```python
from build123d import *

# Parameters (mm, degrees)
SKETCH1_R             = 7.5
BOSS_EXTRUDE1_DEPTH   = 33
M6_TAPPED_HOLE1_D     = 5
M6_TAPPED_HOLE1_DEPTH = 16
M6_TAPPED_HOLE1_TIP   = 1.502151548
M6_TAPPED_HOLE2_D     = 5
M6_TAPPED_HOLE2_DEPTH = 16
M6_TAPPED_HOLE2_TIP   = 1.502151548


with BuildPart() as part:
    # Sketch1 → Boss-Extrude1 (new, symmetric)
    with BuildSketch(Plane.XY):
        Circle(SKETCH1_R)
    extrude(amount=BOSS_EXTRUDE1_DEPTH, both=True)

    # M6 Tapped Hole1
    with Locations(Plane.XY.offset(33)):
        with Locations((0, 0)):
            Hole(M6_TAPPED_HOLE1_D / 2, depth=M6_TAPPED_HOLE1_DEPTH)
            with Locations((0, 0, -(M6_TAPPED_HOLE1_DEPTH + M6_TAPPED_HOLE1_TIP / 2))):  # 118° drill point
                Cone(0, M6_TAPPED_HOLE1_D / 2, M6_TAPPED_HOLE1_TIP, mode=Mode.SUBTRACT)

    # M6 Tapped Hole2
    with Locations(Plane(origin=(0, 0, -33), x_dir=(-1, 0, 0), z_dir=(0, 0, -1))):
        with Locations((0, 0)):
            Hole(M6_TAPPED_HOLE2_D / 2, depth=M6_TAPPED_HOLE2_DEPTH)
            with Locations((0, 0, -(M6_TAPPED_HOLE2_DEPTH + M6_TAPPED_HOLE2_TIP / 2))):  # 118° drill point
                Cone(0, M6_TAPPED_HOLE2_D / 2, M6_TAPPED_HOLE2_TIP, mode=Mode.SUBTRACT)


solid = part.part
```
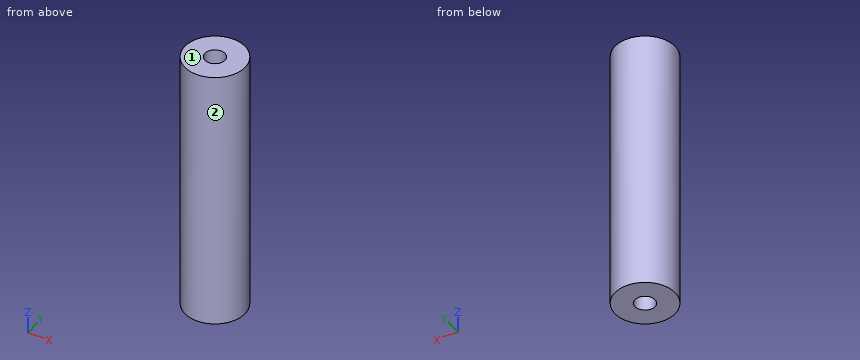
Here's how the part is built. I have some questions about the finished solid (model axes, mm). Face numbers are marked on the shaded views. Coordinates: 2 decimals unless noted, no trailing zeros. Order: outer loops, then holes, each group sorted by start corner. A loop starts at its lowest first (then second) coordinate and runs counter-clockwise, first axis right, second up. Notation, with made-up numbers: M -38,28.5 L 11,28.5 A20 ccw 11,63.5 Z; hole C 68.5,-38.5 d9. An arc over 180 degrees is marked long. Answer as a JSON object with one key per item and string values. Group by question number.
(1) If we mould it in two halves opening along X, with no side actions, what happens to the marked faces 1 and 2? For each: released by +X, released by -X, zero draft, split by the parting line, or undercut.
(2) Suppose I cut it at C-C, the plane x = -6. Please give me the cut outline in (y, z).
(3) Suppose I cut it at D-D, the plane y = 3.75. Please give me the cut outline in (x, z), then the cut area to 3 significant figures.
(4) Suppose I cut it at A-A, the plane z = 8. Please give me the cut outline in (x, y), then the cut area to 3 significant figures.
(5) I need wall thicknesses on probe 1 along Y at (x, z) = (0, -23.5); probe 2 along X at (y, z) = (-0.25, -11); probe 3 along Y at (x, z) = (-4, -20.5). Which ranges of each line are inside material? Lowest first, please.
(6) Suppose I cut it at B-B, the plane z = -27. Please give me the cut outline in (x, y).
(7) For pin 1 (6 mm diameter, centred on x = -5, z = -9.5, fed in from +Y); pin 2 (4.5 mm diameter, centred on x = 0, y = 0, fed in from +Z); pin 3 (2 mm diameter, centred on y = -4.5, z = -15.5, fed in from -X), each with a flat end and sliding along its axis, tell me the tip position at first contact or that it passes through.
Values found:
{
 "1": {"face 1": "zero draft", "face 2": "split by the parting line"},
 "2": {"outline": "M -4.5,-33 L 4.5,-33 L 4.5,33 L -4.5,33 Z"},
 "3": {"outline": "M -6.5,-33 L 6.5,-33 L 6.5,33 L -6.5,33 Z", "area": "857 mm^2"},
 "4": {"outline": "C 0,0 d15", "area": "177 mm^2"},
 "5": {"probe 1": "y = -7.5 to -2.5, 2.5 to 7.5", "probe 2": "x = -7.5 to 7.5", "probe 3": "y = -6.34 to 6.34"},
 "6": {"outline": "C 0,0 d15; hole C 0,0 d5"},
 "7": {"pin 1": "stops at y = 7.23", "pin 2": "stops at z = 16.85", "pin 3": "stops at x = -6.63"}
}
